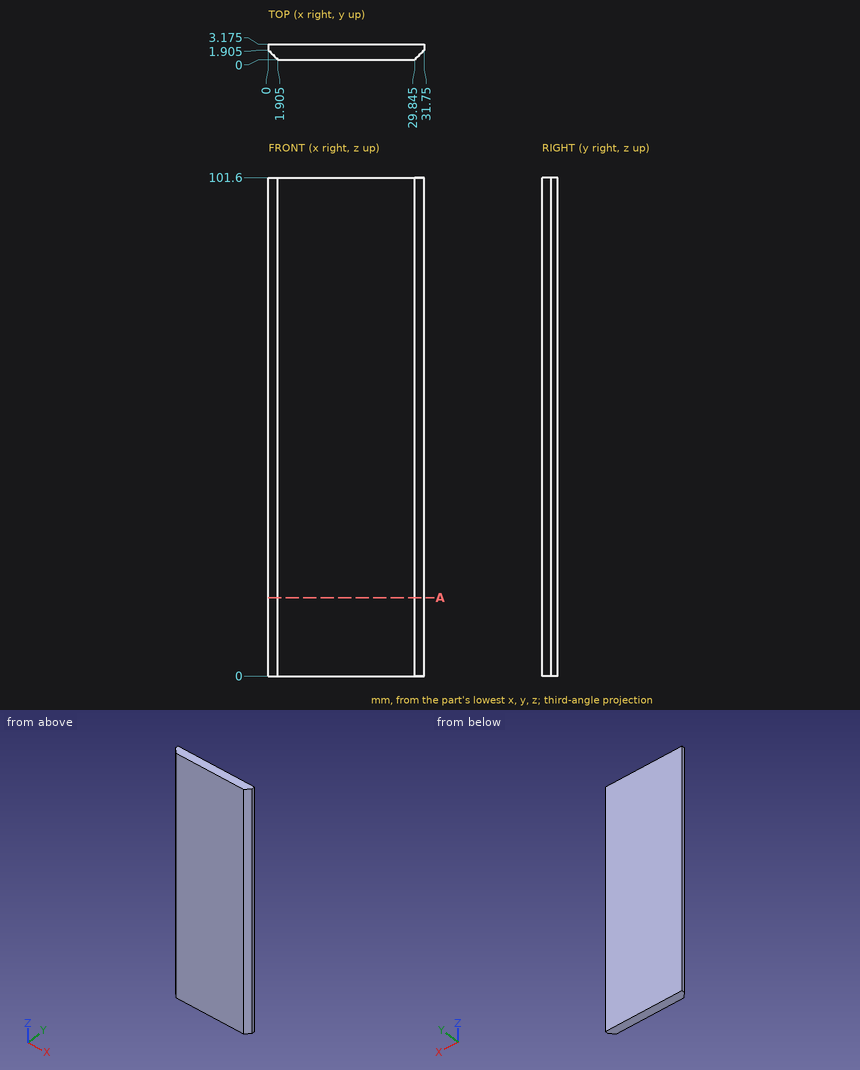
For this review, use the dimensioned drawing (mm, ordinates from the lowest corner) and the shaded views. Coordinates: 2 decimals unless noted, no trailing zeros. Write each loop counter-clockwise with the first axis right and the second up, starting at its lowest first coordinate (ties: lowest second). Pieces come first, ordered by that corner, then holes. Notation, with made-up numbers: (51, 48.5) - (101, 48.5) arc R15 ccw to (101, 66.5) - close; hole circle Ø10 at (-33, 40). An arc over 180 degrees is marked (long way). Answer in a Markdown table with one row per item. Add a question column.
Q1. Clearance check with a flat-ended pin moving along its axis: pin 1 (8 mm diameter, centred on x = 15, z = 20, fed in from -Y). State where the tip first meets the part, or that it passes through.
Q2. Consider section A-A on z = 16. Give the boundary of the cut face in (x, y) (3 decimals), then the cut area to 3 significant figures.
Q3. To check wall thickness, follow line 1 along X through (y, z) = (0.4, 78) (3 decimals); line 2 along X through (y, z) = (1.35, 59.5) (3 decimals); line 3 along Y through (x, z) = (1, 27) (3 decimals). State the ranges of each line that lie inside material, in increasing order. Write a range as from..to.
Answers below:
| question | item | result |
|---|---|---|
| 1 | pin 1 | y = 0 |
| 2 | outline | (0, 1.905) - (1.905, 0) - (29.845, 0) - (31.75, 1.905) - (31.75, 3.175) - (0, 3.175) - close |
| 2 | area | 97.2 mm² |
| 3 | line 1 | 1.505..30.245 |
| 3 | line 2 | 0.555..31.195 |
| 3 | line 3 | 0.905..3.175 |
